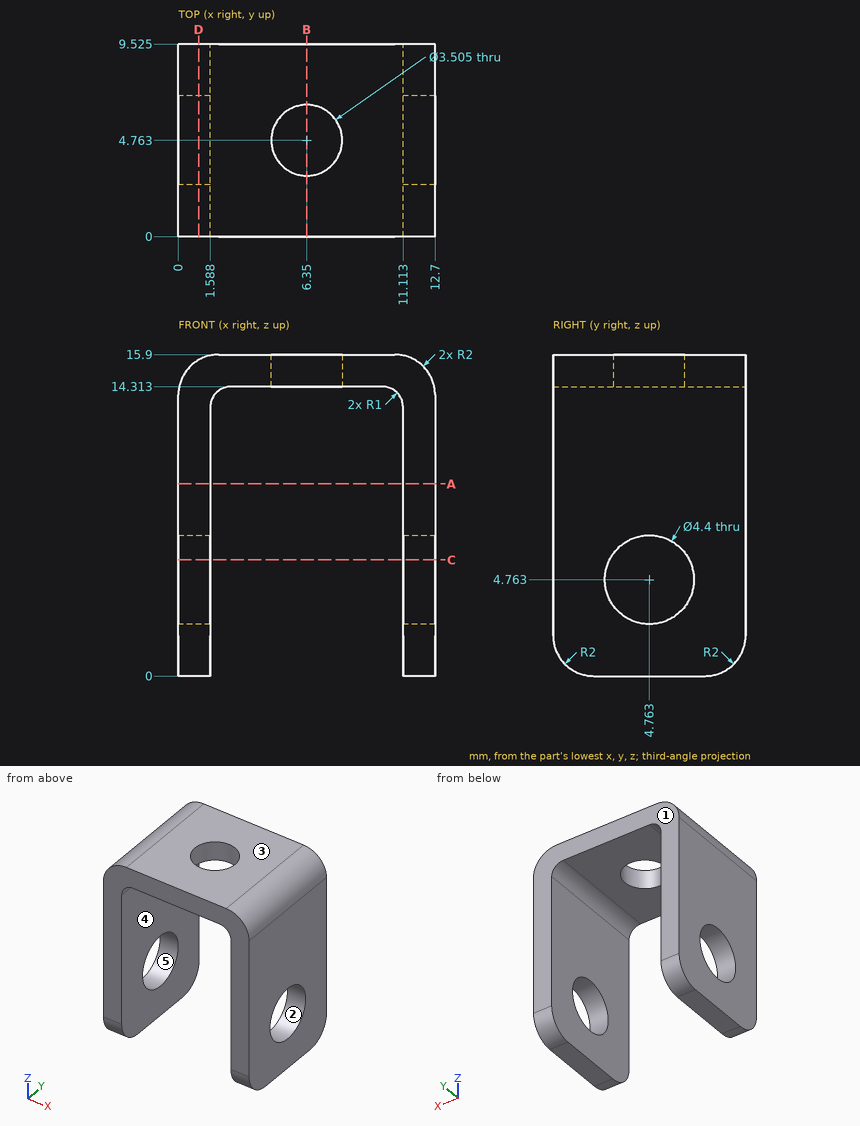
Job drawing, mm, ordinate dimensions from the low corner. One solid piece. A direction names the side the tool comes from. Coordinates: 2 decimals unless noted, no trailing zeros. Loops run counter-clockwise (first coordinate to the right, second up) from the corner with the lowest first, then second, coordinate; pieces in that order, holes last. Notation, with made-up numbers: (-28.5, 3) - (-20.5, 3) arc R20 ccw to (-20.5, 23) - close; hole circle Ø5 at (43.5, 42.5). An arc over 180 degrees is marked (long way). Write item = value, one per line. Start each with the question number.
Q1. Cut at D-D, the plane x = 1. List the corners of the cut face in (y, z) (1 decimal), then the cut area to 3 significant figures.
Q2. Cut at C-C, the plane z = 5.75. List the corners of the cut face in (x, y) (1 decimal).
Q3. Which spindle directions (+Z, -Z, +X, -X, +Y, -Y) get a long thin tool onto all of the face, cutting with end or side? Do the marked faces 4 and 5. Say none if no direction does.
Q4. Drill centre lines: L1, parallel to X at y = 5.75, z = 12.25; L2, parallel to Y at x = 6.35, z = 14.7 (1 decimal); L3, parallel to Z at x = 9.5, y = 2.5. Where is each one in solid material? Low to high.
Q5. Cut at A-A, the plane z = 9.5. List the corners of the cut face in (x, y) (1 decimal).
Q6. Flat gauge pins, fed straight in: pin 1 Ø1.5 at (x, y) = (11, 1) entering from -Z; pin 2 Ø4 at (x, y) = (7, 4.5) entering from -Z. Where does each tip first touch, or does it go through?
Q7. Cut at B-B, the plane x = 6.35. List the corners of the cut face in (y, z) (1 decimal).
Q8. Pull direction Y, two halves, no side cores. Call the marked faces 1, 2 and 3: pulls with the +Y half, pulls with the -Y half, needs draft (parallel to the pull), parting line crosses it, or undercut.
Computed:
q1.outline = (0, 2) arc R2 ccw to (2, 0) - (7.5, 0) arc R2 ccw to (9.5, 2) - (9.5, 15.6) - (0, 15.6) - close; hole circle Ø4.4 at (4.8, 4.8)
q1.area = 132 mm²
q2.outline = (0, 0) - (1.6, 0) - (1.6, 2.8) - (0, 2.8) - close; (0, 6.7) - (1.6, 6.7) - (1.6, 9.5) - (0, 9.5) - close; (11.1, 0) - (12.7, 0) - (12.7, 2.8) - (11.1, 2.8) - close; (11.1, 6.7) - (12.7, 6.7) - (12.7, 9.5) - (11.1, 9.5) - close
q3.face_4 = -Z, +Y, -Y
q3.face_5 = +X, -X
q4.L1 = 0 to 1.59, 11.11 to 12.7
q4.L2 = 0 to 3, 6.5 to 9.5
q4.L3 = 14.31 to 15.9
q5.outline = (0, 0) - (1.6, 0) - (1.6, 9.5) - (0, 9.5) - close; (11.1, 0) - (12.7, 0) - (12.7, 9.5) - (11.1, 9.5) - close
q6.pin_1 = 0.02
q6.pin_2 = 14.31
q7.outline = (0, 14.3) - (3, 14.3) - (3, 15.9) - (0, 15.9) - close; (6.5, 14.3) - (9.5, 14.3) - (9.5, 15.9) - (6.5, 15.9) - close
q8.face_1 = pulls with the +Y half
q8.face_2 = undercut
q8.face_3 = needs draft
